Geometry check sheet. Reference: the model listing, model coordinates, mm. Give positions to 0.01 mm unless a question says otherwise; leave off trailing zeros. Write each loop counter-clockwise with the first axis right and the second up, starting at its lowest first coordinate (ties: lowest second). Pieces come first, ordered by that corner, then holes. Notation, with made-up numbers: (68.25, 67) - (100.25, 67) arc R10 ccw to (100.25, 79) - close; hole circle Ø3 at (-3, -38). An arc over 180 degrees is marked (long way). Write item = value, one per line. Start each with the question number.
(1) Section check C-C, the plane z = 724.5. Enter the section's corners in (x, y) (3 decimals), plus the area to 3 significant figures.
(2) Section check B-B, the plane x = -176.5. Enter the section's corners in (y, z), plus the area to 3 significant figures.
(3) Thickness scan on L1, parallel to X at y = 12.5, z = 962; L2, parallel to Z at x = -396.5, y = 10.5 (3 decimals); L3, parallel to Z at x = -149, y = 11.75. Record the ranges inside material, lowest first.
(4) Section check D-D, the plane y = 11.7. Give the number of separate pieces and of enclosed holes in the cut face, plus the area to 3 significant figures.
(5) Depth check by flat-ended pin: pin 1 Ø10.5 at (x, z) = (-396.5, 962) entering from -Y. Enter the tip coordinate at first touch or a pass-through.
(6) Section check A-A, the plane z = -695. Enter the section's corners in (x, y), plus the area to 3 significant figures.
```python
from build123d import *

# Parameters (mm, degrees)
CROQUIS1_W                 = 630
CROQUIS1_H                 = 1500
CROQUIS1_W_2               = 590
CROQUIS1_H_2               = 1460
SALIENTE_EXTRUIR1_DEPTH    = 20
CROQUIS2_R                 = 5
CORTAR_EXTRUIR1_DEPTH      = 15
REDONDEO1_R                = 2
CORTAR_EXTRUIR2_DEPTH      = 605
CORTAR_EXTRUIR2_DEPTH_BACK = 15
CROQUIS5_R                 = 5
CROQUIS5_R_2               = 3.75
SALIENTE_EXTRUIR2_DEPTH    = 15
ESCALA1_SCALE              = 1.3


with BuildPart() as part:
    # Croquis1 → Saliente-Extruir1 (new body)
    with BuildSketch(Plane(origin=(0, 0, 0), x_dir=(1, 0, 0), z_dir=(0, 1, 0))):
        Rectangle(CROQUIS1_W, CROQUIS1_H)
        Rectangle(CROQUIS1_W_2, CROQUIS1_H_2, mode=Mode.SUBTRACT)
    extrude(amount=SALIENTE_EXTRUIR1_DEPTH)

    # Croquis2 → Cortar-Extruir1 (cut)
    with BuildSketch(Plane.XZ):
        with Locations((-305, 740)):
            Circle(CROQUIS2_R)
        with Locations((305, 740)):
            Circle(CROQUIS2_R)
        with Locations((305, -740)):
            Circle(CROQUIS2_R)
        with Locations((-305, -740)):
            Circle(CROQUIS2_R)
    extrude(amount=-CORTAR_EXTRUIR1_DEPTH, mode=Mode.SUBTRACT)

    # Redondeo1
    redondeo1_edges = [part.edges().sort_by_distance(p)[0] for p in [
        (-315, 20, 0),
        (295, 20, 0),
        (0, 20, 750),
        (0, 20, -730),
        (-295, 20, 0),
        (0, 20, 730),
        (315, 20, 0),
        (0, 20, -750),
    ]]
    fillet(redondeo1_edges, radius=REDONDEO1_R)

    # Croquis4 → Cortar-Extruir2 (cut, two sides)
    with BuildSketch(Plane.ZY.offset(-295)) as cortar_extruir2_sk:
        with BuildLine():
            Line((600, 12.75), (100, 12.75))
            Line((100, 12.75), (100, 5.25))
            Line((100, 5.25), (600, 5.25))
            ThreePointArc((600, 5.25), (603.75, 9), (600, 12.75))
        make_face()
        with BuildLine():
            Line((100, 5.25), (100, 12.75))
            ThreePointArc((100, 12.75), (96.25, 9), (100, 5.25))
        make_face()
    extrude(amount=CORTAR_EXTRUIR2_DEPTH, mode=Mode.SUBTRACT)
    extrude(cortar_extruir2_sk.sketch, amount=-CORTAR_EXTRUIR2_DEPTH_BACK, mode=Mode.SUBTRACT)

    # Croquis5 → Saliente-Extruir2 (add)
    with BuildSketch(Plane.ZY.offset(-295)):
        with Locations((-596.25, 9)):
            Circle(CROQUIS5_R)
        with Locations((-596.25, 9)):
            Circle(CROQUIS5_R_2, mode=Mode.SUBTRACT)
    saliente_extruir2 = extrude(amount=SALIENTE_EXTRUIR2_DEPTH)

    # Simetría1: Saliente-Extruir2 across plane
    add(saliente_extruir2.mirror(Plane(origin=(0, 0, 0), x_dir=(0, 0, 1), z_dir=(1, 0, 0))))


with BuildPart() as part_1:
    # Escala1: scaled about (0, 0, 0)
    add(part.part.scale(ESCALA1_SCALE))


solid = part_1.part
```
Model answer:
q1.outline = (-409.5, 0) - (-383.5, 0) - (-383.5, 6.825) - (-403, 6.825) - (-403, 16.575) - (-383.5, 16.575) - (-383.5, 23.4) arc R2.6 ccw to (-386.1, 26) - (-406.9, 26) arc R2.6 ccw to (-409.5, 23.4) - close; (383.5, 0) - (409.5, 0) - (409.5, 23.4) arc R2.6 ccw to (406.9, 26) - (386.1, 26) arc R2.6 ccw to (383.5, 23.4) - (383.5, 16.575) - (403, 16.575) - (403, 6.825) - (383.5, 6.825) - close
q1.area = 966 mm²
q2.outline = (0, -975) - (23.4, -975) arc R2.6 ccw to (26, -972.4) - (26, -951.6) arc R2.6 ccw to (23.4, -949) - (0, -949) - close; (0, 949) - (23.4, 949) arc R2.6 ccw to (26, 951.6) - (26, 972.4) arc R2.6 ccw to (23.4, 975) - (0, 975) - close
q2.area = 1,350 mm²
q3.L1 = -409.5 to -403, -390 to 390, 403 to 409.5
q3.L2 = -975 to -968.5, -955.5 to 125.275, 784.725 to 955.5, 968.5 to 975
q3.L3 = -975 to -949, 949 to 975
q4.separate_pieces = 1
q4.enclosed_holes = 5
q4.area = 115,000 mm²
q5.pin_1 = 19.5
q6.outline = (-409.5, 0) - (-383.5, 0) - (-383.5, 23.4) arc R2.6 ccw to (-386.1, 26) - (-406.9, 26) arc R2.6 ccw to (-409.5, 23.4) - close; (383.5, 0) - (409.5, 0) - (409.5, 23.4) arc R2.6 ccw to (406.9, 26) - (386.1, 26) arc R2.6 ccw to (383.5, 23.4) - close
q6.area = 1,350 mm²
